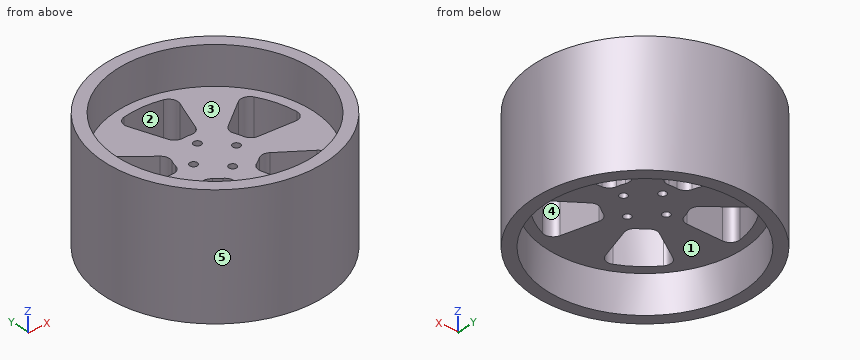
```python
from build123d import *

# Parameters (mm, degrees)
SKETCH1_R           = 72.5
SKETCH1_R_2         = 64.5
BOSS_EXTRUDE1_DEPTH = 40
SKETCH4_R           = 64.5
BOSS_EXTRUDE3_DEPTH = 15
CUT_EXTRUDE1_DEPTH  = 15
SKETCH6_R           = 2.5
CUT_EXTRUDE2_DEPTH  = 30


with BuildPart() as part:
    # Sketch1 → Boss-Extrude1 (new, symmetric)
    with BuildSketch(Plane.XY):
        Circle(SKETCH1_R)
        Circle(SKETCH1_R_2, mode=Mode.SUBTRACT)
    extrude(amount=BOSS_EXTRUDE1_DEPTH, both=True)

    # Sketch4 → Boss-Extrude3 (add, symmetric)
    with BuildSketch(Plane.XY):
        Circle(SKETCH4_R)
    extrude(amount=BOSS_EXTRUDE3_DEPTH, both=True)

    # Sketch3 → Cut-Extrude1 (cut, symmetric)
    with BuildSketch(Plane.XY):
        with BuildLine():
            Line((8.942342186, 26.255693464), (17.100089792, 48.668920804))
            ThreePointArc((17.100089792, 48.668920804), (16.728172015, 53.596235201), (12.784464921, 56.573469548))
            ThreePointArc((12.784464921, 56.573469548), (0, 58), (-12.784464921, 56.573469548))
            ThreePointArc((-12.784464921, 56.573469548), (-16.728172015, 53.596235201), (-17.100089792, 48.668920804))
            Line((-17.100089792, 48.668920804), (-8.942342186, 26.255693464))
            ThreePointArc((-8.942342186, 26.255693464), (-6.454448371, 23.201362532), (-2.608568259, 22.348274467))
            ThreePointArc((-2.608568259, 22.348274467), (0, 22.5), (2.608568259, 22.348274467))
            ThreePointArc((2.608568259, 22.348274467), (6.454448371, 23.201362532), (8.942342186, 26.255693464))
        make_face()
        with BuildLine():
            Line((22.207312654, 16.618128287), (41.002675921, 31.302675452))
            ThreePointArc((41.002675921, 31.302675452), (45.803759299, 32.471584512), (49.853949939, 29.640912191))
            ThreePointArc((49.853949939, 29.640912191), (55.161277945, 17.922985674), (57.755183787, 5.323414851))
            ThreePointArc((57.755183787, 5.323414851), (56.142338174, 0.652710511), (51.571112622, -1.223628199))
            Line((51.571112622, -1.223628199), (27.733984064, -0.391217328))
            ThreePointArc((27.733984064, -0.391217328), (24.060341259, 1.031070133), (22.060563983, 4.425100764))
            ThreePointArc((22.060563983, 4.425100764), (21.398771617, 6.952882373), (20.448380136, 9.386892446))
            ThreePointArc((20.448380136, 9.386892446), (20.071272788, 13.308160497), (22.207312654, 16.618128287))
        make_face()
        with BuildLine():
            Line((22.667216205, -15.985125354), (42.44113714, -29.322803436))
            ThreePointArc((42.44113714, -29.322803436), (45.036452074, -33.527692304), (43.595900456, -38.254378356))
            ThreePointArc((43.595900456, -38.254378356), (34.091544633, -46.922985674), (22.910201686, -53.283418234))
            ThreePointArc((22.910201686, -53.283418234), (17.969701185, -53.19283792), (14.772610647, -49.42516462))
            Line((14.772610647, -49.42516462), (8.198202609, -26.49747907))
            ThreePointArc((8.198202609, -26.49747907), (8.415660309, -22.564126145), (11.025610093, -19.613411791))
            ThreePointArc((11.025610093, -19.613411791), (13.225168177, -18.202882373), (15.246362198, -16.546855886))
            ThreePointArc((15.246362198, -16.546855886), (18.859177151, -14.976467017), (22.667216205, -15.985125354))
        make_face()
        with BuildLine():
            Line((-8.198202609, -26.49747907), (-14.772610647, -49.42516462))
            ThreePointArc((-14.772610647, -49.42516462), (-17.969701185, -53.19283792), (-22.910201686, -53.283418234))
            ThreePointArc((-22.910201686, -53.283418234), (-34.091544633, -46.922985674), (-43.595900456, -38.254378356))
            ThreePointArc((-43.595900456, -38.254378356), (-45.036452074, -33.527692304), (-42.44113714, -29.322803436))
            Line((-42.44113714, -29.322803436), (-22.667216205, -15.985125354))
            ThreePointArc((-22.667216205, -15.985125354), (-18.859177151, -14.976467017), (-15.246362198, -16.546855886))
            ThreePointArc((-15.246362198, -16.546855886), (-13.225168177, -18.202882373), (-11.025610093, -19.613411791))
            ThreePointArc((-11.025610093, -19.613411791), (-8.415660309, -22.564126145), (-8.198202609, -26.49747907))
        make_face()
        with BuildLine():
            Line((-27.733984064, -0.391217328), (-51.571112622, -1.223628199))
            ThreePointArc((-51.571112622, -1.223628199), (-56.142338174, 0.652710511), (-57.755183787, 5.323414851))
            ThreePointArc((-57.755183787, 5.323414851), (-55.161277945, 17.922985674), (-49.853949939, 29.640912191))
            ThreePointArc((-49.853949939, 29.640912191), (-45.803759299, 32.471584512), (-41.002675921, 31.302675452))
            Line((-41.002675921, 31.302675452), (-22.207312654, 16.618128287))
            ThreePointArc((-22.207312654, 16.618128287), (-20.071272788, 13.308160497), (-20.448380136, 9.386892446))
            ThreePointArc((-20.448380136, 9.386892446), (-21.398771617, 6.952882373), (-22.060563983, 4.425100764))
            ThreePointArc((-22.060563983, 4.425100764), (-24.060341259, 1.031070133), (-27.733984064, -0.391217328))
        make_face()
    extrude(amount=CUT_EXTRUDE1_DEPTH, both=True, mode=Mode.SUBTRACT)

    # Sketch6 → Cut-Extrude2 (cut)
    with BuildSketch(Plane.XY.offset(15)):
        with Locations((0, 14)):
            Circle(SKETCH6_R)
        with Locations((14, 0)):
            Circle(SKETCH6_R)
        with Locations((0, -14)):
            Circle(SKETCH6_R)
        with Locations((-14, 0)):
            Circle(SKETCH6_R)
    extrude(amount=-CUT_EXTRUDE2_DEPTH, mode=Mode.SUBTRACT)


solid = part.part
```
Could you check a few things on this model? Use its own coordinates, in mm. Face numbers are marked on the shaded views. A direction names the side the tool comes from. Give positions to 0.01 mm unless a question says otherwise; leave off trailing zeros. Write each loop counter-clockwise with the first axis right and the second up, starting at its lowest first coordinate (ties: lowest second). Pieces come first, ordered by that corner, then holes. Notation, with made-up numbers: (31.25, -19.75) -> (56.25, -19.75) arc R15 ccw to (56.25, -13.75) -> close; hole circle Ø6 at (-33, -29). An arc over 180 degrees is marked (long way). Write each question's results on one line, items separated by ' | '.
1. I want a section at D-D, the plane y = -47. Write out the boundary of the cut face in (x, z), then the cut area to 3 significant figures.
Check sheet entries:
outline: (-55.2, -40) -> (-44.17, -40) -> (-44.17, -15) -> (-33.99, -15) -> (-33.99, 15) -> (-44.17, 15) -> (-44.17, 40) -> (-55.2, 40) -> close; (-14.08, -15) -> (14.08, -15) -> (14.08, 15) -> (-14.08, 15) -> close; (33.99, -15) -> (44.17, -15) -> (44.17, -40) -> (55.2, -40) -> (55.2, 40) -> (44.17, 40) -> (44.17, 15) -> (33.99, 15) -> close | area: 3,220 mm²
2. On a 3-axis mill with a long thin cutter (end or side, diameter ignored), from which of +Z, -Z, +X, -X, +Y, -Y can I reach the whole of each face in a straight line? I mean the marked faces 1, 2 and 3. Say none if no direction works.
Check sheet entries:
face 1: -Z | face 2: +Z, -Z | face 3: +Z
3. I want a section at B-B, the plane y = 45.5. Write out the boundary of the cut face in (x, z).
Check sheet entries:
outline: (-56.44, -40) -> (-45.72, -40) -> (-45.72, -15) -> (-15.95, -15) -> (-15.95, 15) -> (-45.72, 15) -> (-45.72, 40) -> (-56.44, 40) -> close; (15.95, -15) -> (45.72, -15) -> (45.72, -40) -> (56.44, -40) -> (56.44, 40) -> (45.72, 40) -> (45.72, 15) -> (15.95, 15) -> close
4. Will these pins go through, and if not, where does the flat tip stop? pin 1 Ø4 at (x, y) = (-25, 40) entering from -Z; pin 2 Ø10 at (x, z) = (-9, 18) entering from -Y; pin 3 Ø4 at (x, z) = (-10, -28) entering from -Y; pin 4 Ø3 at (x, y) = (14, 0) entering from +Z.
Check sheet entries:
pin 1: stops at z = -15 | pin 2: stops at y = -72.39 | pin 3: stops at y = -72.06 | pin 4: passes through
5. I need wall thicknesses on L1, parallel to Y at x = 0, z = 7; L2, parallel to X at y = 7, z = 2; L3, parallel to Z at x = 28.5, y = 51.5. Which ranges of each line are inside material? Lowest first, please.
Check sheet entries:
L1: y = -72.5 to -16.5, -11.5 to 11.5, 16.5 to 22.5, 58 to 72.5 | L2: x = -72.16 to -57.58, -21.38 to 21.38, 57.58 to 72.16 | L3: z = -15 to 15
6. If we mould it in two halves opening along X, with no side actions, what happens to the marked faces 4 and 5? For each: released by +X, released by -X, zero draft, split by the parting line, or undercut.
Check sheet entries:
face 4: undercut | face 5: split by the parting line
7. I want a section at A-A, the plane x = 0. Write out the boundary of the cut face in (y, z), then the cut area to 4 significant figures.
Check sheet entries:
outline: (-72.5, -40) -> (-64.5, -40) -> (-64.5, -15) -> (-16.5, -15) -> (-16.5, 15) -> (-64.5, 15) -> (-64.5, 40) -> (-72.5, 40) -> close; (-11.5, -15) -> (11.5, -15) -> (11.5, 15) -> (-11.5, 15) -> close; (16.5, -15) -> (22.5, -15) -> (22.5, 15) -> (16.5, 15) -> close; (58, -15) -> (64.5, -15) -> (64.5, -40) -> (72.5, -40) -> (72.5, 40) -> (64.5, 40) -> (64.5, 15) -> (58, 15) -> close | area: 3,785 mm²
8. I want a section at C-C, the plane z = 20.5. Write out the boundary of the cut face in (x, y), then the cut area to 3 significant figures.
Check sheet entries:
outline: circle Ø145 at (0, 0); hole circle Ø129 at (0, 0) | area: 3,440 mm²
